Part print with two shaded views. Sizes in mm from the minimum x, y, z corner. A direction names the side the tool comes from. Round coordinates to 2 decimals unless told otherwise and drop trailing zeros. Write each loop counter-clockwise with the first axis right and the second up, starting at its lowest first coordinate (ties: lowest second). Pieces come first, ordered by that corner, then holes. Notation, with made-up numbers: M 5.5,36 L 33.5,36 A22 cw 33.5,63 Z; hole C 51,-24 d2. An arc over 180 degrees is marked long. One line per question, with ' | ' between items. Start each with the question number.
1) Tool access for the marked faces 1, 2, 3 and 4: list every direction of +Z, -Z, +X, -X, +Y, -Y with a clear straight run to the whole face (end or side of a thin tool).
2) Saw through at A-A (z = 1.75). List the corners of the cut face in (x, y).
3) Saw through at B-B (x = 16.5). List the corners of the cut face in (y, z).
4) Saw through at C-C (y = 15.5). List the corners of the cut face in (x, z), plus the area to 3 significant figures.
5) Wall check: probe 1 along X at (y, z) = (40, 1.55); probe 2 along X at (y, z) = (16, 1.3); probe 3 along Y at (x, z) = (12.5, 3.95). Give the ranges that are in metal, low to high. Write a range as [from, to].
6) Drop flat-ended pins along their axis: pin 1 Ø2.5 at (y, z) = (14.5, 2) entering from +X; pin 2 Ø1.5 at (y, z) = (33.5, 1) entering from -X; pin 3 Ø1.6 at (y, z) = (2, 1.5) entering from +X. Give the stop position or say it passes through.
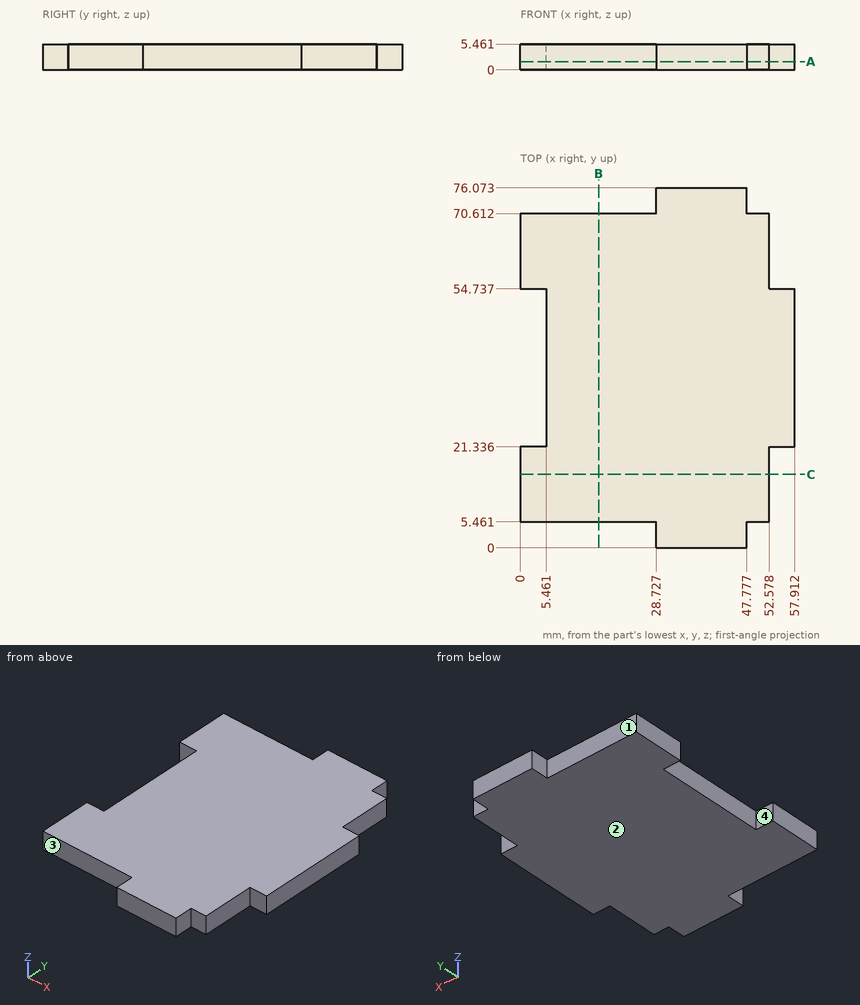
Answer key:
1) face 1: +Z, -Z, -X, +Y | face 2: -Z, +X, -X, +Y, -Y | face 3: +Z, -Z, -X, -Y | face 4: +Z, -Z, -X
2) outline: M 0,5.46 L 28.73,5.46 L 28.73,0 L 47.78,0 L 47.78,5.46 L 52.58,5.46 L 52.58,21.34 L 57.91,21.34 L 57.91,54.74 L 52.58,54.74 L 52.58,70.61 L 47.78,70.61 L 47.78,76.07 L 28.73,76.07 L 28.73,70.61 L 0,70.61 L 0,54.74 L 5.46,54.74 L 5.46,21.34 L 0,21.34 Z
3) outline: M 5.46,0 L 70.61,0 L 70.61,5.46 L 5.46,5.46 Z
4) outline: M 0,0 L 52.58,0 L 52.58,5.46 L 0,5.46 Z | area: 287 mm2
5) probe 1: x = [5.46, 57.91] | probe 2: x = [0, 52.58] | probe 3: y = [5.46, 70.61]
6) pin 1: stops at x = 52.58 | pin 2: stops at x = 5.46 | pin 3: stops at x = 47.78
